Check sheet for the modelled part. Datum: model origin and axes. Units: mm. Face numbers are marked on the shaded views. Round coordinates to 2 decimals unless told otherwise and drop trailing zeros. Order: outer loops, then holes, each group sorted by start corner. A loop starts at its lowest first (then second) coordinate and runs counter-clockwise, first axis right, second up.
```python
from build123d import *

# Parameters (mm, degrees)
BOSS_EXTRUDE1_DEPTH = 15
CUT_EXTRUDE1_DEPTH  = 73.629551255
SKETCH8_R           = 1.75
CUT_EXTRUDE2_DEPTH  = 73.629551255
CUT_EXTRUDE4_DEPTH  = 73.629551255


with BuildPart() as part:
    # Sketch3 → Boss-Extrude1 (new body)
    with BuildSketch(Plane.XY):
        Polygon((-60.537407798, -1.859852476), (69.462592202, -1.859852476), (69.462592202, -2.859852476), (-59.537407798, -2.859852476), (-59.537407798, -15.859852476), (69.462592202, -15.859852476), (69.462592202, -16.859852476), (-60.537407798, -16.859852476), align=None)
    extrude(amount=-BOSS_EXTRUDE1_DEPTH)

    # Sketch6 → Cut-Extrude1 (cut, through all)
    with BuildSketch(Plane(origin=(0, -1.859852476, 0), x_dir=(1, 0, 0), z_dir=(0, 1, 0))):
        Polygon((-60.537407798, 12), (-10.537407798, 0), (-10.537407798, -10.064923469), (-60.537407798, -10.064923469), align=None)
    extrude(amount=-CUT_EXTRUDE1_DEPTH, mode=Mode.SUBTRACT)

    # Sketch8 → Cut-Extrude2 (cut, through all)
    with BuildSketch(Plane(origin=(0, -1.859852476, 0), x_dir=(1, 0, 0), z_dir=(0, 1, 0))):
        with Locations(Location((-50.537407798, 12.7, 0), (0, 0, 270))):
            Circle(SKETCH8_R)
    extrude(amount=-CUT_EXTRUDE2_DEPTH, mode=Mode.SUBTRACT)

    # Sketch12 → Cut-Extrude4 (cut, through all)
    with BuildSketch(Plane.XZ.offset(16.859852476)):
        with BuildLine():
            Line((53.415401878, -12.5), (-36.584598122, -12.5))
            ThreePointArc((-36.584598122, -12.5), (-38.334598122, -10.75), (-36.584598122, -9))
            Line((-36.584598122, -9), (53.415401878, -9))
            ThreePointArc((53.415401878, -9), (55.165401878, -10.75), (53.415401878, -12.5))
        make_face()
    extrude(amount=-CUT_EXTRUDE4_DEPTH, mode=Mode.SUBTRACT)


solid = part.part
```
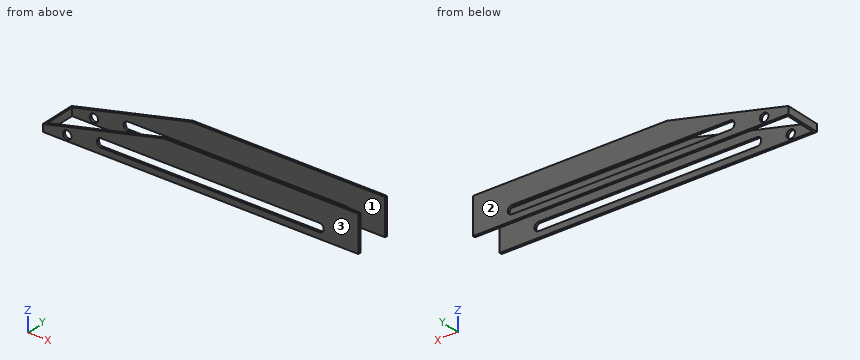
Item 1: Sectioned sample at B-B (x = 58.5). Record the cut outline in (y, z), and give its area (3 significant figures).
Answer:
outline: (-16.86, -15) - (-15.86, -15) - (-15.86, 0) - (-16.86, 0) - close; (-2.86, -15) - (-1.86, -15) - (-1.86, 0) - (-2.86, 0) - close
area: 30.0 mm2
Item 2: Go/stop test with flat-tipped pins: P1, Ø4, axis at y = -14.5, z = -3.5, coming from the +X side; P2, Ø3, axis at x = -50.54, z = -12.7, coming from the +Y side; P3, Ø1, axis at y = -11.5, z = -13.5, coming from the +X side. Record where each tip stops, or that it passes through.
Answer:
P1: stops at x = 69.46
P2: passes through
P3: stops at x = -59.54
Item 3: Sectioned sample at D-D (y = -10.5). Record the cut outline in (x, z).
Answer:
outline: (-60.54, -15) - (-59.54, -15) - (-59.54, -11.76) - (-60.54, -12) - close
Item 4: Release check for a two-part mould opening along Y. For the marked faces 1, 2 and 3 record: released by +Y, released by -Y, zero draft, split by the parting line, or undercut.
Answer:
face 1: undercut
face 2: released by +Y
face 3: released by -Y
Item 5: Scan lines: line 1 along Y through (x, z) = (15, -14); line 2 along X through (y, z) = (-16.55, -12.7); line 3 along Z through (x, y) = (1.5, -16). Record each from-to range of solid material in increasing order.
Answer:
line 1: y = -16.86 to -15.86, -2.86 to -1.86
line 2: x = -60.54 to -52.29, -48.79 to 69.46
line 3: z = -15 to -12.5, -9 to 0
Item 6: Sectioned sample at C-C (z = -2.25). Record the cut outline in (x, y), and give its area (3 significant figures).
Answer:
outline: (-19.91, -16.86) - (69.46, -16.86) - (69.46, -15.86) - (-19.91, -15.86) - close; (-19.91, -2.86) - (69.46, -2.86) - (69.46, -1.86) - (-19.91, -1.86) - close
area: 179 mm2
Item 7: Sectioned sample at A-A (x = 22). Record the cut outline in (y, z).
Answer:
outline: (-16.86, -15) - (-15.86, -15) - (-15.86, -12.5) - (-16.86, -12.5) - close; (-16.86, -9) - (-15.86, -9) - (-15.86, 0) - (-16.86, 0) - close; (-2.86, -15) - (-1.86, -15) - (-1.86, -12.5) - (-2.86, -12.5) - close; (-2.86, -9) - (-1.86, -9) - (-1.86, 0) - (-2.86, 0) - close
